from build123d import *

# Parameters (mm, degrees)
SKETCH1_W           = 5.08
SKETCH1_H           = 1.044000004
BOSS_EXTRUDE1_DEPTH = 3.175
EXTRUDE_THIN1_DEPTH = 2.54


with BuildPart() as part:
    # Sketch1 → Boss-Extrude1 (new body, symmetric)
    with BuildSketch(Plane(origin=(0, 0, 0), x_dir=(0, 0, -1), z_dir=(1, 0, 0))):
        with Locations((0, 0.522000002)):
            Rectangle(SKETCH1_W, SKETCH1_H)
    extrude(amount=BOSS_EXTRUDE1_DEPTH, both=True)

    # Sketch2 → Extrude-Thin1 (add, symmetric)
    with BuildSketch(Plane(origin=(0, 0, 0), x_dir=(0, 0, -1), z_dir=(1, 0, 0))):
        Polygon((-2.54, 0.522000002), (-3.429, 0.522000002), (-3.429, 0), (-4.318, 0), (-4.318, 0.127), (-3.556, 0.127), (-3.556, 0.649000002), (-2.54, 0.649000002), align=None)
    extrude_thin1 = extrude(amount=EXTRUDE_THIN1_DEPTH, both=True)

    # Mirror1: Extrude-Thin1 across plane
    add(extrude_thin1.mirror(Plane.XY))


solid = part.part
The model under review builds one solid part; all positions refer to its coordinate system, in mm. Give positions to 0.01 mm unless a question says otherwise; leave off trailing zeros. Order: outer loops, then holes, each group sorted by start corner. A loop starts at its lowest first (then second) coordinate and runs counter-clockwise, first axis right, second up. Notation, with made-up numbers: M 27.25,64.25 L 72.25,64.25 A21 ccw 72.25,83.25 Z; hole C 83.5,80.5 d4. An arc over 180 degrees is marked long. Answer in a Markdown table with one row per item. Add a question column.
1. Add section D-D on y = 0.9. State the section outline as (x, z) points (3 decimals), plus the area to 3 significant figures.
2. Add section C-C on z = 2.75. State the section outline as (x, y) points, plus the area to 3 significant figures.
3. Mouldability with a two-part tool opening along Z and no side actions: class faces 1 (the flat face through (0, 0.3, 2.54)), 2 (the flat face through (-3.175, 0.5, 0)) as released by +Z, released by -Z, zero draft, split by the parting line, or undercut.
4. Add section B-B on x = 0.5. State the section outline as (y, z) points.
5. Add section A-A on y = 0.4. State the section outline as (x, z) points (3 decimals), plus the area to 3 significant figures.
6. To check wall thickness, follow line 1 along Z through (x, y) = (-3, 0.8). State the ranges of the line that lie inside material, in increasing order.
7. For pin 1 Ø0.6 at (x, y) = (-1, 0.5) entering from -Z; pin 2 Ø0.8 at (x, z) = (0.5, 4) entering from +Y; pin 3 Ø1 at (x, z) = (-2.5, 3) entering from +Y; pin 4 Ø0.5 at (x, z) = (0.5, 3) entering from +Y, all flat-tipped, find the tip position at first contact; note any pin that passes through.
The answers:
| question | item | result |
|---|---|---|
| 1 | outline | M -3.175,-2.54 L 3.175,-2.54 L 3.175,2.54 L -3.175,2.54 Z |
| 1 | area | 32.3 mm2 |
| 2 | outline | M -2.54,0.52 L 2.54,0.52 L 2.54,0.65 L -2.54,0.65 Z |
| 2 | area | 0.645 mm2 |
| 3 | face 1 | undercut |
| 3 | face 2 | zero draft |
| 4 | outline | M 0,-4.32 L 0.13,-4.32 L 0.13,-3.56 L 0.65,-3.56 L 0.65,-2.54 L 1.04,-2.54 L 1.04,2.54 L 0.65,2.54 L 0.65,3.56 L 0.13,3.56 L 0.13,4.32 L 0,4.32 L 0,3.43 L 0.52,3.43 L 0.52,2.54 L 0,2.54 L 0,-2.54 L 0.52,-2.54 L 0.52,-3.43 L 0,-3.43 Z |
| 5 | outline | M -3.175,-2.54 L 3.175,-2.54 L 3.175,2.54 L -3.175,2.54 Z; M -2.54,-3.556 L 2.54,-3.556 L 2.54,-3.429 L -2.54,-3.429 Z; M -2.54,3.429 L 2.54,3.429 L 2.54,3.556 L -2.54,3.556 Z |
| 5 | area | 33.5 mm2 |
| 6 | line 1 | -2.54 to 2.54 |
| 7 | pin 1 | z = -3.56 |
| 7 | pin 2 | y = 0.13 |
| 7 | pin 3 | y = 1.04 |
| 7 | pin 4 | y = 0.65 |
